```python
from build123d import *

# Parameters (mm, degrees)
BOSS_EXTRUDE1_DEPTH      = 5.08
BOSS_EXTRUDE1_DEPTH_BACK = 5.08
SKETCH1_W                = 6.35
SKETCH1_H                = 6.35
SKETCH1_R                = 1.905
SKETCH2_R                = 1.27
BOSS_EXTRUDE2_DEPTH      = 6.35
BOSS_EXTRUDE3_START      = 6.35
SKETCH3_R                = 1.27
BOSS_EXTRUDE3_DEPTH      = 6.35
SCALE1_SCALE             = 8


with BuildPart() as part:
    # Sketch1 → Boss-Extrude1 (new, two sides: drawn at the far end of the back side and taken through both)
    with BuildSketch(Plane.XY.offset(-BOSS_EXTRUDE1_DEPTH_BACK)):
        Rectangle(SKETCH1_W, SKETCH1_H)
        Circle(SKETCH1_R, mode=Mode.SUBTRACT)
    extrude(amount=BOSS_EXTRUDE1_DEPTH + BOSS_EXTRUDE1_DEPTH_BACK)

    # Sketch2 → Boss-Extrude2 (add)
    with BuildSketch(Plane.ZY.offset(3.175)):
        Circle(SKETCH2_R)
    extrude(amount=BOSS_EXTRUDE2_DEPTH)

    # Sketch3 → Boss-Extrude3 (add)
    with BuildSketch(Plane(origin=(3.175, 0, 0), x_dir=(0, 0, -1), z_dir=(1, 0, 0)).offset(BOSS_EXTRUDE3_START)):
        with Locations(Location((0, 0, 0), (0, 0, 180))):
            Circle(SKETCH3_R)
    extrude(amount=-BOSS_EXTRUDE3_DEPTH)


with BuildPart() as part_1:
    # Scale1: scaled about (0, 0, 0)
    add(part.part.scale(SCALE1_SCALE))


solid = part_1.part
```
Here's how the part is built. I have some questions about the finished solid (model axes, mm). A direction names the side the tool comes from. Coordinates: 2 decimals unless noted, no trailing zeros. Loops run counter-clockwise (first coordinate to the right, second up) from the corner with the lowest first, then second, coordinate; pieces in that order, holes last. Notation, with made-up numbers: (23, 60) - (60, 60) arc R18 ccw to (60, 84) - close; hole circle Ø7 at (75, 75). An arc over 180 degrees is marked (long way). Return JSON: item names as keys, results as strings. Group by question number.
Item 1: I need wall thicknesses on line 1 (Y direction, x = 0, z = -17); line 2 (X direction, y = -20, z = 28); line 3 (X direction, y = -13.5, z = -13.5). Which ranges of each line are inside material? Lowest first, please. Write a range as from..to.
Item 2: If we section it at C-C on z = 0: Write out the boundary of the cut face in (x, y), and give its area (3 significant figures).
Item 3: We'd pull the mould along X, two halves only. Please class faces 4 (the face through (25.4, -6, -10)), 5 (the face through (-3.3, -14.88, -0.57)), 6 (the face through (-25.4, -6, -10)), 7 (the face through (11, -11, -40.64)): +X half, -X half, draft (parallel to the pull), parting line (faces both ways), or undercut.
Item 4: If we section it at A-A on x = 0: Write out the boundary of the cut face in (y, z), and give its area (3 significant figures).
Item 5: On a 3-axis mill with a long thin cutter (end or side, diameter ignored), from which of +Z, -Z, +X, -X, +Y, -Y can I reach the whole of each face in a straight line? I mean faces 1 (the face through (-50.444, 10.074, -1.323)), 2 (the face through (51.156, -10.074, -1.323)), 3 (the face through (11, -11, 40.64)). Say none if no direction works.
Item 6: Will these pins go through, and if not, where does the flat tip stop? P1, Ø1, axis at y = 15.5, z = 22, coming from the -X side; P2, Ø2, axis at x = 40.5, y = 2.5, coming from the -Z side; P3, Ø8, axis at x = -56, z = 15, coming from the -Y side; P4, Ø8, axis at x = 41.5, z = 5, coming from the +Y side.
Item 7: If we section it at B-B on y = 0: Write out the boundary of the cut face in (x, z).
Item 8: If we section it at D-D on x = -46.5: Write out the boundary of the cut face in (y, z).
Calculated:
{
 "1": {"line 1": "y = -25.4..-15.24, 15.24..25.4", "line 2": "x = -25.4..25.4", "line 3": "x = -25.4..-7.07, 7.07..25.4"},
 "2": {"outline": "(-76.2, -10.16) - (-25.4, -10.16) - (-25.4, -25.4) - (25.4, -25.4) - (25.4, -10.16) - (76.2, -10.16) - (76.2, 10.16) - (25.4, 10.16) - (25.4, 25.4) - (-25.4, 25.4) - (-25.4, 10.16) - (-76.2, 10.16) - close; hole circle Ø30.48 at (0, 0)", "area": "3,920 mm^2"},
 "3": {"face 4": "+X half", "face 5": "undercut", "face 6": "-X half", "face 7": "draft"},
 "4": {"outline": "(-25.4, -40.64) - (-15.24, -40.64) - (-15.24, 40.64) - (-25.4, 40.64) - close; (15.24, -40.64) - (25.4, -40.64) - (25.4, 40.64) - (15.24, 40.64) - close", "area": "1,650 mm^2"},
 "5": {"face 1": "-X", "face 2": "+X", "face 3": "+Z, +X, -X, +Y, -Y"},
 "6": {"P1": "stops at x = -25.4", "P2": "stops at z = -10.05", "P3": "passes through", "P4": "stops at y = 10.11"},
 "7": {"outline": "(-76.2, -10.16) - (-25.4, -10.16) - (-25.4, -40.64) - (-15.24, -40.64) - (-15.24, 40.64) - (-25.4, 40.64) - (-25.4, 10.16) - (-76.2, 10.16) - close; (15.24, -40.64) - (25.4, -40.64) - (25.4, -10.16) - (76.2, -10.16) - (76.2, 10.16) - (25.4, 10.16) - (25.4, 40.64) - (15.24, 40.64) - close"},
 "8": {"outline": "circle Ø20.32 at (0, 0)"}
}
